from build123d import *

# Parameters (mm, degrees)
F0_W     = 597
F0_H     = 600
F0_R     = 11.15
F0_R_2   = 2.75
F0_R_3   = 3
F0_R_4   = 8
F0_R_5   = 8.5
F0_R_6   = 3.3
F0_W_2   = 32.3
F0_H_2   = 32.3
F0_R_7   = 5.5
F0_W_3   = 32
F0_H_3   = 32
F1_DEPTH = 1.6
F2_R     = 3
F2_R_2   = 8.5
F2_R_3   = 3.3
F2_W     = 34
F2_H     = 34
F3_DEPTH = 5
F4_R     = 3.3
F4_W     = 34.3
F4_H     = 34.3
F4_R_2   = 3
F4_R_3   = 8.5
F5_DEPTH = 5


with BuildPart() as f1:
    # F0 (on Top) → F1 (new body)
    with BuildSketch(Plane.XY):
        Rectangle(F0_W, F0_H)
        with Locations((-239.0813, -167.15)):
            Circle(F0_R, mode=Mode.SUBTRACT)
        with Locations((-95.05, -252.5)):
            Circle(F0_R, mode=Mode.SUBTRACT)
        with Locations((-239.0813, -117.15)):
            Circle(F0_R, mode=Mode.SUBTRACT)
        with Locations((-239.0813, -37.15)):
            Circle(F0_R, mode=Mode.SUBTRACT)
        with Locations((-35.05, -78.5)):
            Circle(F0_R_2, mode=Mode.SUBTRACT)
        with Locations((-118.4, -73.5)):
            Circle(F0_R_3, mode=Mode.SUBTRACT)
        with Locations((-95.05, -52)):
            Circle(F0_R_4, mode=Mode.SUBTRACT)
        with Locations((-118.4, -30.5)):
            Circle(F0_R_3, mode=Mode.SUBTRACT)
        with Locations((-73.4, -73.5)):
            Circle(F0_R_3, mode=Mode.SUBTRACT)
        with Locations((-35.05, -59)):
            Circle(F0_R_5, mode=Mode.SUBTRACT)
        with Locations((-35.05, -39.5)):
            Circle(F0_R_2, mode=Mode.SUBTRACT)
        with Locations((-73.4, -30.5)):
            Circle(F0_R_3, mode=Mode.SUBTRACT)
        with Locations((34.95, -252.5)):
            Circle(F0_R, mode=Mode.SUBTRACT)
        Polygon((159.5, -247.236544), (159.5, -257.763456), (153.763456, -263.5), (143.236544, -263.5), (137.5, -257.763456), (137.5, -247.236544), (143.236544, -241.5), (153.763456, -241.5), align=None, mode=Mode.SUBTRACT)
        with Locations((13.45, -175.35)):
            Circle(F0_R_3, mode=Mode.SUBTRACT)
        with Locations((34.95, -152)):
            Circle(F0_R_4, mode=Mode.SUBTRACT)
        with Locations((56.45, -175.35)):
            Circle(F0_R_3, mode=Mode.SUBTRACT)
        with Locations((94.95, -178.5)):
            Circle(F0_R_2, mode=Mode.SUBTRACT)
        with Locations((94.95, -159)):
            Circle(F0_R_5, mode=Mode.SUBTRACT)
        with Locations((13.45, -130.35)):
            Circle(F0_R_3, mode=Mode.SUBTRACT)
        with Locations((56.45, -130.35)):
            Circle(F0_R_3, mode=Mode.SUBTRACT)
        with Locations((94.95, -139.5)):
            Circle(F0_R_2, mode=Mode.SUBTRACT)
        with Locations((100.7, -3)):
            Circle(F0_R_6, mode=Mode.SUBTRACT)
        with Locations((164.7, -3)):
            Circle(F0_R_6, mode=Mode.SUBTRACT)
        with Locations((-244.5, 97)):
            Circle(F0_R_6, mode=Mode.SUBTRACT)
        with Locations((-180.5, 97)):
            Circle(F0_R_6, mode=Mode.SUBTRACT)
        with Locations((-212.5, 129)):
            Rectangle(F0_W_2, F0_H_2, mode=Mode.SUBTRACT)
        with Locations((-244.5, 161)):
            Circle(F0_R_6, mode=Mode.SUBTRACT)
        with Locations((-180.5, 161)):
            Circle(F0_R_6, mode=Mode.SUBTRACT)
        with Locations((-212.5, 204.15)):
            Circle(F0_R_7, mode=Mode.SUBTRACT)
        with Locations((132.55, 29.15)):
            Rectangle(F0_W_3, F0_H_3, mode=Mode.SUBTRACT)
        with Locations((100.7, 61)):
            Circle(F0_R_6, mode=Mode.SUBTRACT)
        with Locations((132.7, 104.15)):
            Circle(F0_R_7, mode=Mode.SUBTRACT)
        with Locations((164.7, 61)):
            Circle(F0_R_6, mode=Mode.SUBTRACT)
    extrude(amount=F1_DEPTH)

    # F2 (on Top) → F3 (join)
    with BuildSketch(Plane.XY):
        with BuildLine():
            ThreePointArc((75.45, -197.35), (77.57132, -196.47132), (78.45, -194.35))
            Line((78.45, -194.35), (78.45, -99.742772))
            ThreePointArc((78.45, -99.742772), (78.80056, -98.335481), (79.770311, -97.257084))
            Line((79.770311, -97.257084), (185.379689, -25.892192))
            ThreePointArc((185.379689, -25.892192), (186.34944, -24.813795), (186.7, -23.406504))
            Line((186.7, -23.406504), (186.7, 83.3))
            ThreePointArc((186.7, 83.3), (185.82132, 85.42132), (183.7, 86.3))
            Line((183.7, 86.3), (80.599617, 86.3))
            ThreePointArc((80.599617, 86.3), (78.994692, 85.834603), (77.887718, 84.582809))
            Line((77.887718, 84.582809), (-8.2619, -97.540223))
            ThreePointArc((-8.2619, -97.540223), (-8.477089, -98.165651), (-8.55, -98.823032))
            Line((-8.55, -98.823032), (-8.55, -194.35))
            ThreePointArc((-8.55, -194.35), (-7.67132, -196.47132), (-5.55, -197.35))
            Line((-5.55, -197.35), (75.45, -197.35))
        make_face()
        with Locations((13.45, -175.35)):
            Circle(F2_R, mode=Mode.SUBTRACT)
        with Locations((13.45, -130.35)):
            Circle(F2_R, mode=Mode.SUBTRACT)
        with Locations((34.95, -152)):
            Circle(F2_R_2, mode=Mode.SUBTRACT)
        with Locations((56.45, -175.35)):
            Circle(F2_R, mode=Mode.SUBTRACT)
        with Locations((56.45, -130.35)):
            Circle(F2_R, mode=Mode.SUBTRACT)
        with Locations((100.7, -3)):
            Circle(F2_R_3, mode=Mode.SUBTRACT)
        with Locations((164.7, -3)):
            Circle(F2_R_3, mode=Mode.SUBTRACT)
        with Locations((132.55, 29.15)):
            Rectangle(F2_W, F2_H, mode=Mode.SUBTRACT)
        with Locations((100.7, 61)):
            Circle(F2_R_3, mode=Mode.SUBTRACT)
        with Locations((164.7, 61)):
            Circle(F2_R_3, mode=Mode.SUBTRACT)
    extrude(amount=-F3_DEPTH)

    # F4 (on face) → F5 (join)
    with BuildSketch(Plane(origin=(0, 0, 0), x_dir=(1, 0, 0), z_dir=(0, 0, -1))):
        with BuildLine():
            ThreePointArc((-137.4, 96.975185), (-139.52132, 96.096505), (-140.4, 93.975185))
            Line((-140.4, 93.975185), (-140.4, 3.76251))
            ThreePointArc((-140.4, 3.76251), (-140.783333, 2.295182), (-141.835368, 1.202837))
            Line((-141.835368, 1.202837), (-265.064632, -74.122613))
            ThreePointArc((-265.064632, -74.122613), (-266.116667, -75.214958), (-266.5, -76.682286))
            Line((-266.5, -76.682286), (-266.5, -180))
            ThreePointArc((-266.5, -180), (-265.62132, -182.12132), (-263.5, -183))
            Line((-263.5, -183), (-160.230076, -183))
            ThreePointArc((-160.230076, -183), (-158.731359, -182.598817), (-157.633483, -181.502565))
            Line((-157.633483, -181.502565), (-51.803407, 1.383094))
            ThreePointArc((-51.803407, 1.383094), (-51.502606, 2.107771), (-51.4, 2.885659))
            Line((-51.4, 2.885659), (-51.4, 93.975185))
            ThreePointArc((-51.4, 93.975185), (-52.27868, 96.096505), (-54.4, 96.975185))
            Line((-54.4, 96.975185), (-137.4, 96.975185))
        make_face()
        with Locations((-244.5, -161)):
            Circle(F4_R, mode=Mode.SUBTRACT)
        with Locations((-180.5, -161)):
            Circle(F4_R, mode=Mode.SUBTRACT)
        with Locations((-212.5, -129)):
            Rectangle(F4_W, F4_H, mode=Mode.SUBTRACT)
        with Locations((-244.5, -97)):
            Circle(F4_R, mode=Mode.SUBTRACT)
        with Locations((-180.5, -97)):
            Circle(F4_R, mode=Mode.SUBTRACT)
        with Locations((-118.4, 30.5)):
            Circle(F4_R_2, mode=Mode.SUBTRACT)
        with Locations((-118.4, 73.5)):
            Circle(F4_R_2, mode=Mode.SUBTRACT)
        with Locations((-95.05, 52)):
            Circle(F4_R_3, mode=Mode.SUBTRACT)
        with Locations((-73.4, 30.5)):
            Circle(F4_R_2, mode=Mode.SUBTRACT)
        with Locations((-73.4, 73.5)):
            Circle(F4_R_2, mode=Mode.SUBTRACT)
    extrude(amount=F5_DEPTH)


solid = f1.part
The listing builds one solid part. Answer for the finished solid, in the listing's coordinates (mm). A direction names the side the tool comes from. Give positions to 0.01 mm unless a question says otherwise; leave off trailing zeros. Write each loop counter-clockwise with the first axis right and the second up, starting at its lowest first coordinate (ties: lowest second). Pieces come first, ordered by that corner, then holes.
1) Section D-D (x = 229.5) is taken. Write down the section's boundary in (y, z), and give its area (3 significant figures).
2) A tool of negligible diameter and unlimited length cuts with its end or side. For faces 4 (the face through (-213.9, 112.6, 0)), 5 (the face through (-160, 41, -5)), 6 (the face through (35.416, -5.204, -2.465)), from which of +Z, -Z, +X, -X, +Y, -Y can it reach the whole face along a straight path? Write none if from no direction.
3) Find the intervals of material crossed by L1, parallel to X at y = 139.5, z = -4.5; L2, parallel to Z at x = 249, y = -249; L3, parallel to X at y = 161, z = -1, in increasing order.
4) Section B-B (y = 129) is taken. Write down the section's boundary in (x, z).
5) Section A-A (z = -2.5) is taken. Count the separate pieces of the cut face and the enclosed holes in it, and give its area (3 significant figures).
6) For a pull along Y with two mould halves and no side action, classify faces 1 (the face through (-4, 4, 0)), 2 (the face through (131.8, -62.1, -2.5)), 3 (the face through (98.87, -166.54, 0.79)) as pulls with the +Y half, pulls with the -Y half, needs draft (parallel to the pull), parting line crosses it, or undercut.
7) Given P1, Ø5, axis at x = 84, y = -222.5, coming from the -Z side; P2, Ø1.5, axis at y = 132.5, z = -3.5, coming from the -X side; P3, Ø2.5, axis at y = 132, z = -3, coming from the +X side, each flat-ended and moving along its own axis, determine where each tip first touches the part or whether it passes through.
8) Section C-C (x = 34.95) is taken. Write down the section's boundary in (y, z).
Response:
1. outline: (-300, 0) - (300, 0) - (300, 1.6) - (-300, 1.6) - close
1. area: 960 mm2
2. face 4: -Z
2. face 5: -Z, +X, -X, +Y, -Y
2. face 6: -Z, +Y
3. L1: x = -266.5 to -229.65, -195.35 to -133.33
3. L2: z = 0 to 1.6
3. L3: x = -266.5 to -247.8, -241.2 to -183.8, -177.2 to -145.77
4. outline: (-298.5, 0) - (-266.5, 0) - (-266.5, -5) - (-229.65, -5) - (-229.65, 0) - (-228.65, 0) - (-228.65, 1.6) - (-298.5, 1.6) - close; (-196.35, 0) - (-195.35, 0) - (-195.35, -5) - (-127.25, -5) - (-127.25, 0) - (298.5, 0) - (298.5, 1.6) - (-196.35, 1.6) - close
5. separate pieces: 2
5. enclosed holes: 20
5. area: 62,800 mm2
6. face 1: needs draft
6. face 2: pulls with the -Y half
6. face 3: undercut
7. P1: stops at z = 0
7. P2: stops at x = -266.5
7. P3: stops at x = -128.26
8. outline: (-300, 0) - (-263.65, 0) - (-263.65, 1.6) - (-300, 1.6) - close; (-241.35, 0) - (-197.35, 0) - (-197.35, -5) - (-160.5, -5) - (-160.5, 0) - (-160, 0) - (-160, 1.6) - (-241.35, 1.6) - close; (-144, 0) - (-143.5, 0) - (-143.5, -5) - (-6.19, -5) - (-6.19, 0) - (300, 0) - (300, 1.6) - (-144, 1.6) - close
